Verification items for the finished model (mm, model axes). A direction names the side the tool comes from. Round coordinates to 2 decimals unless told otherwise and drop trailing zeros. Order: outer loops, then holes, each group sorted by start corner. A loop starts at its lowest first (then second) coordinate and runs counter-clockwise, first axis right, second up. Notation, with made-up numbers: (57, -31.5) -> (111, -31.5) arc R20 cw to (111, -2.5) -> close; hole circle Ø1 at (49, -28.75). An arc over 180 degrees is marked (long way). Write item = value, one per line. Start each with the question number.
from build123d import *

# Parameters (mm, degrees)
SKETCH1_R           = 8
BOSS_EXTRUDE1_DEPTH = 15
SKETCH2_R           = 1.65
CUT_EXTRUDE1_DEPTH  = 23
SKETCH3_R           = 8
SKETCH3_R_2         = 4
BOSS_EXTRUDE2_DEPTH = 14
FILLET1_R           = 0.5
CHAMFER1_SIZE       = 0.5


with BuildPart() as part:
    # Sketch1 → Boss-Extrude1 (new body, symmetric)
    with BuildSketch(Plane.XY):
        Polygon((-17, 11.5), (-7, 11.5), (-7, 10.5), (7, 10.5), (7, 11.5), (17, 11.5), (17, 5.5), (15, 3.5), (15, -6.5), (10, -6.5), (6, -10.5), (-6, -10.5), (-10, -6.5), (-15, -6.5), (-15, 3.5), (-17, 5.5), align=None)
        Circle(SKETCH1_R, mode=Mode.SUBTRACT)
    extrude(amount=BOSS_EXTRUDE1_DEPTH, both=True)

    # Sketch2 → Cut-Extrude1 (cut, through all)
    with BuildSketch(Plane(origin=(0, 11.5, 0), x_dir=(1, 0, 0), z_dir=(0, 1, 0))):
        with Locations((-12, 9)):
            Circle(SKETCH2_R)
        with Locations((-12, -9)):
            Circle(SKETCH2_R)
        with Locations((12, -9)):
            Circle(SKETCH2_R)
        with Locations((12, 9)):
            Circle(SKETCH2_R)
    extrude(amount=-CUT_EXTRUDE1_DEPTH, mode=Mode.SUBTRACT)

    # Sketch3 → Boss-Extrude2 (add, symmetric)
    with BuildSketch(Plane.XY):
        Circle(SKETCH3_R)
        Circle(SKETCH3_R_2, mode=Mode.SUBTRACT)
    extrude(amount=BOSS_EXTRUDE2_DEPTH, both=True)

    # Fillet1
    fillet1_edges = [part.edges().sort_by_distance(p)[0] for p in [
        (-13.65, 11.5, -9),
        (-13.65, 11.5, 9),
        (10.35, 11.5, 9),
        (10.35, 11.5, -9),
    ]]
    fillet(fillet1_edges, radius=FILLET1_R)

    # Chamfer1
    chamfer1_edges = [part.edges().sort_by_distance(p)[0] for p in [
        (-17, 11.5, 0),
        (-7, 11.5, 0),
        (7, 11.5, 0),
        (17, 11.5, 0),
        (15, -6.5, 0),
        (-15, -6.5, 0),
    ]]
    chamfer(chamfer1_edges, length=CHAMFER1_SIZE)


solid = part.part
(1) Cross-section at D-D (z = -9). Give the number of separate pieces and of enclosed holes in the cut face, and give its area (3 significant figures).
(2) Depth check by flat-ended pin: pin 1 (1 mm diameter, centred on y = -1, z = 8.5, fed in from -X); pin 2 (10.5 mm diameter, centred on y = -3, z = -3.5, fed in from +X); pin 3 (4.5 mm diameter, centred on x = -12, z = 9, fed in from -Y). Enter the tip coordinate at first touch or a pass-through.
(3) Scan lines: line 1 along Y through (x, z) = (0, -14.4); line 2 along Z through (x, y) = (-13, -1.5); line 3 along Z through (x, y) = (-12, -1.5). Record each from-to range of solid material in increasing order. Write a range as from..to.
(4) Cross-section at B-B (z = 4.5). Enter the section's corners in (x, y), and give its area (3 significant figures).
(5) Cross-section at A-A (y = 0). Enter the section's corners in (x, z).
(6) Draft check along X on faces 4 (the flat face through (-4, 8, 15)), 5 (the flat face through (-17, 8, 0)), 6 (the flat face through (16, 4.5, 0.2)), 7 (the flat face through (0, 10.5, 0)). Enter one of: +X half, -X half, draft (parallel to the pull), parting line (faces both ways), or undercut.
(7) Cross-section at C-C (x = -1). Enter the section's corners in (y, z).
(8) Set-up check for faces 1 (the flat face through (15, -1, 0)), 2 (the flat face through (-4, -2, 14)), 3 (the flat face through (-12, -6.5, 0)): record each of +Z, -Z, +X, -X, +Y, -Y from which the full face is reachable in a straight line by a thin tool's end or side.
Outcome:
q1.separate_pieces = 3
q1.enclosed_holes = 1
q1.area = 448 mm^2
q2.pin_1 = -15
q2.pin_2 = 15
q2.pin_3 = -6.75
q3.line_1 = -10.5..-8, 8..10.5
q3.line_2 = -15..-10.31, -7.69..7.69, 10.31..15
q3.line_3 = -15..-10.65, -7.35..7.35, 10.65..15
q4.outline = (-17, 5.5) -> (-15, 3.5) -> (-15, -6) -> (-14.5, -6.5) -> (-10, -6.5) -> (-6, -10.5) -> (6, -10.5) -> (10, -6.5) -> (14.5, -6.5) -> (15, -6) -> (15, 3.5) -> (17, 5.5) -> (17, 11) -> (16.5, 11.5) -> (7.5, 11.5) -> (7, 11) -> (7, 10.5) -> (-7, 10.5) -> (-7, 11) -> (-7.5, 11.5) -> (-16.5, 11.5) -> (-17, 11) -> close; hole circle Ø8 at (0, 0)
q4.area = 567 mm^2
q5.outline = (-15, -15) -> (-8, -15) -> (-8, -14) -> (-4, -14) -> (-4, 14) -> (-8, 14) -> (-8, 15) -> (-15, 15) -> close; (4, -14) -> (8, -14) -> (8, -15) -> (15, -15) -> (15, 15) -> (8, 15) -> (8, 14) -> (4, 14) -> close; hole circle Ø3.3 at (-12, -9); hole circle Ø3.3 at (-12, 9); hole circle Ø3.3 at (12, -9); hole circle Ø3.3 at (12, 9)
q6.face_4 = draft
q6.face_5 = -X half
q6.face_6 = +X half
q6.face_7 = undercut
q7.outline = (-10.5, -15) -> (-7.94, -15) -> (-7.94, -14) -> (-3.87, -14) -> (-3.87, 14) -> (-7.94, 14) -> (-7.94, 15) -> (-10.5, 15) -> close; (3.87, -14) -> (7.94, -14) -> (7.94, -15) -> (10.5, -15) -> (10.5, 15) -> (7.94, 15) -> (7.94, 14) -> (3.87, 14) -> close
q8.face_1 = +Z, -Z, +X, -Y
q8.face_2 = +Z
q8.face_3 = +Z, -Z, -X, -Y
